Here's how the part is built. I have some questions about the finished solid (model axes, mm). A direction names the side the tool comes from. Coordinates: 2 decimals unless noted, no trailing zeros. Loops run counter-clockwise (first coordinate to the right, second up) from the corner with the lowest first, then second, coordinate; pieces in that order, holes last. Notation, with made-up numbers: (15.5, -9.5) - (20.5, -9.5) arc R26 ccw to (20.5, 19.5) - close; hole circle Ø9 at (17.25, -14). An arc over 180 degrees is marked (long way). Use a Markdown table: item, result.
Autodesk Inventor part; units mm, degrees
ref_plane "YZ Plane" through (0, 0, 0) normal (1, 0, 0) x (0, 1, 0)
ref_plane "XZ Plane" through (0, 0, 0) normal (0, 1, 0) x (-1, 0, 0)
ref_plane "XY Plane" through (0, 0, 0) normal (0, 0, 1) x (1, 0, 0)
sketch "Sketch15" plane through (0, 0, 0) normal (0, 0, 1) x (1, 0, 0)
  line L0 (0, 0) -> (0, 1.4)
  line L1 (0.2309, 1.8) -> (1.5, 1.8)
  line L2 (1.5, 1.8) -> (1.5, 2.5)
  line L3 (1.5, 2.5) -> (1.7, 2.5)
  line L4 (1.7, 2.5) -> (1.7, 1)
  line L5 (1.7, 1) -> (12, 1)
  line L6 (12, 0) -> (0, 0)
  line L7 (0.2309, 1.8) -> (0, 1.4)
  line L8 (12, 1) -> (12, 0)
  dimension "d78" = 0.2
  dimension "d83" = 30
  dimension "d84" = 1
  dimension "d86" = 0.4
  dimension "d87" = 1.8
  dimension "d89" = 1.5
  dimension "d90" = 2.5
  dimension "d115" = 12
revolve "Revolution1" add sketch "Sketch15" angle 360 about axis through (12, 0, 0) along (-1, 0, 0)
thread "Thread2"
sketch "Sketch16" plane through (0, 0, 0) normal (-1, 0, 0) x (0, 0, 1)
  circle A0 centre (0, 0) radius 1.4
  line L0 (0.9238, 1.6) -> (1.8475, 0)
  line L1 (1.8475, 0) -> (0.9238, -1.6)
  line L2 (0.9238, -1.6) -> (-0.9238, -1.6)
  line L3 (-0.9238, -1.6) -> (-1.8475, 0)
  line L4 (-1.8475, 0) -> (-0.9238, 1.6)
  line L5 (-0.9238, 1.6) -> (0.9238, 1.6)
  circle A1 centre (0, 0) radius 2.6573
  dimension "d104" = 3.2
extrude "Extrusion15" cut sketch "Sketch16" against normal up to surface (1.5 mm away) contours A1
chamfer "Chamfer5" distance 0.2 angle 45 1 edges at (12, -1, 0)
properties part number "Bolt"
Q1. Please list where these lines run through material, in increasing order: L1, parallel to X at y = -1.8, z = 1; L2, parallel to X at y = -1, z = -0.3; L3, parallel to Y at x = 10.25, z = 0. Write a range as from..to.
Check values:
| item | result |
|---|---|
| L1 | 1.5..1.7 |
| L2 | 0..1.7 |
| L3 | -1..1 |
Q2. I want a section at B-B, the plane x = 6.5. Write out the boundary of the cut face in (y, z), then the cut area to 3 significant figures.
Check values:
| item | result |
|---|---|
| outline | circle Ø2 at (0, 0) |
| area | 3.14 mm^2 |
Q3. Will these pins go through, and if not, where does the flat tip stop? P1, Ø2, axis at x = 2.5, z = -1.5, coming from the -Y side; P2, Ø3, axis at x = 6.5, y = 0.5, coming from the -Z side; P3, Ø3, axis at x = 5, y = 0.5, coming from the +Z side.
Check values:
| item | result |
|---|---|
| P1 | y = -2.33 |
| P2 | z = -1 |
| P3 | z = 1 |
Q4. Which directions (+Z, -Z, +X, -X, +Y, -Y) give clear straight access to the entire face, cutting with the end or side of a thin tool? Please do faces 1 (the face through (1, -1.6, 0)), 2 (the face through (0.8, -0.79, 1.39)), 3 (the face through (7, 0, -1)), 4 (the face through (1, 1.6, 0)).
Check values:
| item | result |
|---|---|
| face 1 | +Z, -Z, -X, -Y |
| face 2 | +Z, -X, -Y |
| face 3 | +X |
| face 4 | +Z, -Z, -X, +Y |
Q5. I want a section at C-C, the plane z = 2.1. Write out the boundary of the cut face in (x, y).
Check values:
| item | result |
|---|---|
| outline | (1.5, -1.36) - (1.7, -1.36) - (1.7, 1.36) - (1.5, 1.36) - close |
Q6. I want a section at A-A, the plane z = 0. Write out the boundary of the cut face in (x, y).
Check values:
| item | result |
|---|---|
| outline | (0, -1.4) - (0.12, -1.6) - (1.5, -1.6) - (1.5, -2.5) - (1.7, -2.5) - (1.7, -1) - (11.8, -1) - (12, -0.8) - (12, 0.8) - (11.8, 1) - (1.7, 1) - (1.7, 2.5) - (1.5, 2.5) - (1.5, 1.6) - (0.12, 1.6) - (0, 1.4) - close |
